Can you work these out from the model? Positions are in its coordinate system, mm. Face numbers are marked on the shaded views. A direction names the side the tool comes from. Coordinates: 2 decimals unless noted, no trailing zeros. Loops run counter-clockwise (first coordinate to the right, second up) from the corner with the lowest first, then second, coordinate; pieces in that order, holes last.
```python
from build123d import *

# Parameters (mm, degrees)
BOSS_EXTRUDE1_DEPTH                                 = 34
CBORE_FOR_M3_HEX_SOCKET_HEAD_CAP_SCREW1_D           = 3.4
CBORE_FOR_M3_HEX_SOCKET_HEAD_CAP_SCREW1_CBORE_D     = 6.5
CBORE_FOR_M3_HEX_SOCKET_HEAD_CAP_SCREW1_CBORE_DEPTH = 10


with BuildPart() as part:
    # Sketch1 → Boss-Extrude1 (new, symmetric)
    with BuildSketch(Plane.XY):
        Polygon((0, 0), (0, -11.547005384), (20, -11.547005384), align=None)
    extrude(amount=BOSS_EXTRUDE1_DEPTH, both=True)

    # CBORE for M3 Hex Socket Head Cap Screw1 (through all)
    with Locations(Plane(origin=(0, 0, 0), x_dir=(1, 0, 0), z_dir=(0, 1, 0))):
        with Locations((8, -25), (8, 25)):
            CounterBoreHole(CBORE_FOR_M3_HEX_SOCKET_HEAD_CAP_SCREW1_D / 2, CBORE_FOR_M3_HEX_SOCKET_HEAD_CAP_SCREW1_CBORE_D / 2, CBORE_FOR_M3_HEX_SOCKET_HEAD_CAP_SCREW1_CBORE_DEPTH)

    # Chamfer1
    # the kernel refuses this chamfer: 0.5, 0.366025404 mm, written as the material it takes off along each edge
    with BuildSketch(Plane(origin=(0.333333333, -11.21367205, 33.666666667), x_dir=(0.7071067811865475, -0.7071067811865476, 0), z_dir=(-0.5773502691896258, -0.5773502691896257, 0.5773502691896256)), Plane(origin=(0.333333333, -11.21367205, -33.666666667), x_dir=(0.7071067811865474, 0, -0.7071067811865476), z_dir=(-0.5773502691896258, -0.5773502691896257, -0.5773502691896257))) as chamfer1_piece_1:
        Polygon((-0.353553391, -0.204124145), (0.353553391, -0.204124145), (0, 0.40824829), align=None)
    extrude(amount=0.635085296, mode=Mode.SUBTRACT)
    with BuildSketch(Plane(origin=(19.105662433, -11.319334483, 33.666666667), x_dir=(-0.8880738339771186, 0.3250575836718637, 0.3250575836718637), z_dir=(0.25056280708572953, -0.2505628070857271, 0.9351131265310311))) as chamfer1_piece_2:
        Polygon((-0.478383292, 0.07914139), (1.059805709, 0.07914139), (-0.581422417, -0.15828278), align=None)
    extrude(amount=0.652121763, mode=Mode.SUBTRACT)
    with BuildSketch(Plane(origin=(19.105662433, -11.319334483, -33.666666667), x_dir=(0.8880738339771186, -0.3250575836718637, 0.3250575836718637), z_dir=(0.25056280708572953, -0.2505628070857271, -0.9351131265310311))) as chamfer1_piece_3:
        Polygon((-1.059805709, 0.07914139), (0.478383292, 0.07914139), (0.581422417, -0.15828278), align=None)
    extrude(amount=0.652121763, mode=Mode.SUBTRACT)
    with BuildSketch(Plane(origin=(0.311004234, -0.494016936, -33.666666667), x_dir=(0.5773502691896288, -0.5773502691896194, -0.5773502691896291), z_dir=(-0.16369153687076843, 0.6109051323707225, -0.7745966692414806))) as chamfer1_piece_4:
        Polygon((-0.349679369, 0.136409614), (0.516346035, 0.136409614), (-0.166666667, -0.272819228), align=None)
    extrude(amount=0.671995646, mode=Mode.SUBTRACT)
    with BuildSketch(Plane(origin=(0.311004234, -0.494016936, 33.666666667), x_dir=(0.5773502691896286, -0.5773502691896196, 0.5773502691896291), z_dir=(-0.1636915368707684, 0.6109051323707224, 0.7745966692414807))) as chamfer1_piece_5:
        Polygon((-0.349679369, -0.136409614), (0.516346035, -0.136409614), (-0.166666667, 0.272819228), align=None)
    extrude(amount=0.671995646, mode=Mode.SUBTRACT)
    with BuildSketch(Plane(origin=(-1.285841494, -11.547005384, 34), x_dir=(0, -0.02749587661058574, -0.9996219169112968), z_dir=(1, 0, 0)), Plane(origin=(-1.285841494, -11.547005384, -34), x_dir=(0, 0.999621916911297, -0.0274958766105822), z_dir=(1, 0, 0))) as chamfer1_piece_6:
        with BuildLine():
            Line((0.514336598, 0), (-0.028273577, 0.513558897))
            Line((-0.028273577, 0.513558897), (-0.038269797, 0.513283938))
            ThreePointArc((-0.038269797, 0.513283938), (-0.017064614, 0.256698915), (-0.009996219, -0.000274959))
            Line((-0.009996219, -0.000274959), (0.000274959, -0.009996219))
            ThreePointArc((0.000274959, -0.009996219), (0.257248832, -0.002927825), (0.514611556, -0.009996219))
            Line((0.514611556, -0.009996219), (0.514336598, 0))
        make_face()
    extrude(amount=22.571682988, mode=Mode.SUBTRACT)
    with BuildSketch(Plane(origin=(8, -11.547005384, -25), x_dir=(-1, 0, 0), z_dir=(0, 0, 1))) as chamfer1_piece_7:
        with BuildLine():
            Line((2.214142136, 0.014142136), (1.685857864, -0.514142136))
            Line((1.685857864, -0.514142136), (1.675857864, -0.514142136))
            ThreePointArc((1.675857864, -0.514142136), (1.69, -0.257071068), (1.69, 0))
            Line((1.69, 0), (1.7, 0.01))
            ThreePointArc((1.7, 0.01), (1.957071068, 0.01), (2.214142136, 0.024142136))
            Line((2.214142136, 0.024142136), (2.214142136, 0.014142136))
        make_face()
    revolve(axis=Axis((8, -11.547005384, -25), (0, -1, 0)), mode=Mode.SUBTRACT)
    with BuildSketch(Plane(origin=(8, -11.547005384, 25), x_dir=(-1, 0, 0), z_dir=(0, 0, 1))) as chamfer1_piece_8:
        with BuildLine():
            Line((2.214142136, 0.014142136), (1.685857864, -0.514142136))
            Line((1.685857864, -0.514142136), (1.675857864, -0.514142136))
            ThreePointArc((1.675857864, -0.514142136), (1.69, -0.257071068), (1.69, 0))
            Line((1.69, 0), (1.7, 0.01))
            ThreePointArc((1.7, 0.01), (1.957071068, 0.01), (2.214142136, 0.024142136))
            Line((2.214142136, 0.024142136), (2.214142136, 0.014142136))
        make_face()
    revolve(axis=Axis((8, -11.547005384, 25), (0, -1, 0)), mode=Mode.SUBTRACT)
    with BuildSketch(Plane(origin=(0, 1.285841494, -34), x_dir=(-0.027495876610586483, 0, 0.9996219169112968), z_dir=(0, -1, 0))) as chamfer1_piece_9:
        with BuildLine():
            Line((0.514336598, 0), (-0.028273577, -0.513558897))
            Line((-0.028273577, -0.513558897), (-0.038269797, -0.513283938))
            ThreePointArc((-0.038269797, -0.513283938), (-0.017064614, -0.256698915), (-0.009996219, 0.000274959))
            Line((-0.009996219, 0.000274959), (0.000274959, 0.009996219))
            ThreePointArc((0.000274959, 0.009996219), (0.257248832, 0.002927825), (0.514611556, 0.009996219))
            Line((0.514611556, 0.009996219), (0.514336598, 0))
        make_face()
    extrude(amount=14.118688372, mode=Mode.SUBTRACT)
    with BuildSketch(Plane(origin=(21.113571399, -12.189926131, -34), x_dir=(-0.4998109584556428, -0.8656979742248838, -0.027495876610582233), z_dir=(-0.8660254037844419, 0.4999999999999943, 0))) as chamfer1_piece_10:
        with BuildLine():
            Line((0.514336598, 0), (-0.028273577, 0.513558897))
            Line((-0.028273577, 0.513558897), (-0.038269797, 0.513283938))
            ThreePointArc((-0.038269797, 0.513283938), (-0.017064614, 0.256698915), (-0.009996219, -0.000274959))
            Line((-0.009996219, -0.000274959), (0.000274959, -0.009996219))
            ThreePointArc((0.000274959, -0.009996219), (0.257248832, -0.002927825), (0.514611556, -0.009996219))
            Line((0.514611556, -0.009996219), (0.514336598, 0))
        make_face()
    extrude(amount=25.665693756, mode=Mode.SUBTRACT)
    with BuildSketch(Plane(origin=(21.113571399, -12.189926131, 34), x_dir=(-0.4998109584556428, -0.8656979742248838, 0.027495876610582233), z_dir=(-0.8660254037844419, 0.4999999999999943, 0))) as chamfer1_piece_11:
        with BuildLine():
            Line((0.514336598, 0), (-0.028273577, -0.513558897))
            Line((-0.028273577, -0.513558897), (-0.038269797, -0.513283938))
            ThreePointArc((-0.038269797, -0.513283938), (-0.017064614, -0.256698915), (-0.009996219, 0.000274959))
            Line((-0.009996219, 0.000274959), (0.000274959, 0.009996219))
            ThreePointArc((0.000274959, 0.009996219), (0.257248832, 0.002927825), (0.514611556, 0.009996219))
            Line((0.514611556, 0.009996219), (0.514336598, 0))
        make_face()
    extrude(amount=25.665693756, mode=Mode.SUBTRACT)
    with BuildSketch(Plane(origin=(0, -11.547005384, -35.285841494), x_dir=(-0.02749587661058639, 0.9996219169112968, 0), z_dir=(0, 0, 1))) as chamfer1_piece_12:
        with BuildLine():
            Line((0.514336598, 0), (-0.028273577, -0.513558897))
            Line((-0.028273577, -0.513558897), (-0.038269797, -0.513283938))
            ThreePointArc((-0.038269797, -0.513283938), (-0.017064614, -0.256698915), (-0.009996219, 0.000274959))
            Line((-0.009996219, 0.000274959), (0.000274959, 0.009996219))
            ThreePointArc((0.000274959, 0.009996219), (0.257248832, 0.002927825), (0.514611556, 0.009996219))
            Line((0.514611556, 0.009996219), (0.514336598, 0))
        make_face()
    extrude(amount=70.571682988, mode=Mode.SUBTRACT)
    with BuildSketch(Plane(origin=(0, 1.285841494, 34), x_dir=(-0.027495876610586483, 0, -0.9996219169112968), z_dir=(0, -1, 0))) as chamfer1_piece_13:
        with BuildLine():
            Line((0.514336598, 0), (-0.028273577, 0.513558897))
            Line((-0.028273577, 0.513558897), (-0.038269797, 0.513283938))
            ThreePointArc((-0.038269797, 0.513283938), (-0.017064614, 0.256698915), (-0.009996219, -0.000274959))
            Line((-0.009996219, -0.000274959), (0.000274959, -0.009996219))
            ThreePointArc((0.000274959, -0.009996219), (0.257248832, -0.002927825), (0.514611556, -0.009996219))
            Line((0.514611556, -0.009996219), (0.514336598, 0))
        make_face()
    extrude(amount=14.118688372, mode=Mode.SUBTRACT)
    with BuildSketch(Plane(origin=(20, -11.547005384, 35.285841494), x_dir=(-0.9996219169112968, -0.02749587661058555, 0), z_dir=(0, 0, -1))) as chamfer1_piece_14:
        with BuildLine():
            Line((0.514336598, 0), (0.297309717, 0.20540729))
            Line((0.297309717, 0.20540729), (0.292073486, 0.21392679))
            ThreePointArc((0.292073486, 0.21392679), (0.148476438, 0.10299394), (-0.005236231, 0.0085195))
            Line((-0.005236231, 0.0085195), (0.000274959, -0.009996219))
            ThreePointArc((0.000274959, -0.009996219), (0.257248832, -0.002927825), (0.514611556, -0.009996219))
            Line((0.514611556, -0.009996219), (0.514336598, 0))
        make_face()
    extrude(amount=70.571682988, mode=Mode.SUBTRACT)
    with BuildSketch(Plane(origin=(0, 0, 35.285841494), x_dir=(-0.05197283076278021, -0.9986484991539833, 0), z_dir=(0, 0, -1))) as chamfer1_piece_15:
        with BuildLine():
            Line((0.371704143, 0), (0.220983806, -0.464444069))
            Line((0.220983806, -0.464444069), (0.212075392, -0.468987213))
            ThreePointArc((0.212075392, -0.468987213), (0.107882689, -0.233552691), (-0.008908414, -0.004543145))
            Line((-0.008908414, -0.004543145), (0.000519728, 0.009986485))
            ThreePointArc((0.000519728, 0.009986485), (0.185869781, 0.000340281), (0.372223871, 0.009986485))
            Line((0.372223871, 0.009986485), (0.371704143, 0))
        make_face()
    extrude(amount=70.571682988, mode=Mode.SUBTRACT)


solid = part.part
```
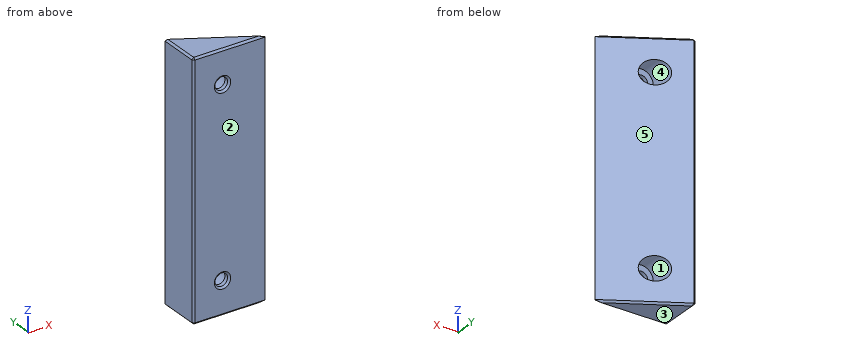
(1) I want a section at C-C on x = 8. Write out the boundary of the cut face in (y, z).
Check values:
outline: (-11.55, -33.5) - (-11.05, -34) - (-5.2, -34) - (-4.62, -33.5) - (-4.62, -28.25) - (-10, -28.25) - (-10, -26.7) - (-11.05, -26.7) - (-11.55, -27.2) - close; (-11.55, -22.8) - (-11.05, -23.3) - (-10, -23.3) - (-10, -21.75) - (-4.62, -21.75) - (-4.62, 21.75) - (-10, 21.75) - (-10, 23.3) - (-11.05, 23.3) - (-11.55, 22.8) - close; (-11.55, 27.2) - (-11.05, 26.7) - (-10, 26.7) - (-10, 28.25) - (-4.62, 28.25) - (-4.62, 33.5) - (-5.2, 34) - (-11.05, 34) - (-11.55, 33.5) - close
(2) Which directions (+Z, -Z, +X, -X, +Y, -Y) give clear straight access to the entire face, cutting with the end or side of a thin tool? Please do the marked faces 1 and 2.
Check values:
face 1: +Y
face 2: +Z, -Z, +X, -X, -Y
(3) I want a section at A-A on y = -8.25. Write out the boundary of the cut face in (x, z).
Check values:
outline: (0, -33.5) - (0.5, -34) - (13.29, -34) - (14.29, -33.5) - (14.29, 33.5) - (13.29, 34) - (0.5, 34) - (0, 33.5) - close; hole circle Ø6.5 at (8, -25); hole circle Ø6.5 at (8, 25)
(4) I'm going to push flat-ended pins straight in: pin 1 (1 mm diameter, centred on x = 6.5, z = -17, fed in from +Y); pin 2 (5 mm diameter, centred on x = 9, z = 24.5, fed in from +Y); pin 3 (4 mm diameter, centred on x = 8, z = 25, fed in from +Y). Where does each tip first touch, or does it pass through?
Check values:
pin 1: stops at y = -3.46
pin 2: stops at y = -5.36
pin 3: stops at y = -10
(5) If I drill on probe 1 along Z at (x, y) = (8, -8); probe 2 along Z at (x, y) = (8, -10.7); probe 3 along X at (y, z) = (-4.75, 25), over which ranges is the centre line in solid material (lowest first)?
Check values:
probe 1: z = -34 to -28.25, -21.75 to 21.75, 28.25 to 34
probe 2: z = -34 to -26.7, -23.3 to 23.3, 26.7 to 34
probe 3: x = 0 to 4.75
(6) I want a section at D-D on y = -3.5. Write out the boundary of the cut face in (x, z).
Check values:
outline: (0, -33.5) - (0.5, -34) - (5.06, -34) - (6.06, -33.5) - (6.06, -27.61) arc R3.25 cw to (6.06, -22.39) - (6.06, 22.39) arc R3.25 cw to (6.06, 27.61) - (6.06, 33.5) - (5.06, 34) - (0.5, 34) - (0, 33.5) - close
(7) If we mould it in two halves opening along X, with no side actions, what happens to the marked faces 3, 4 and 5? For each: released by +X, released by -X, zero draft, split by the parting line, or undercut.
Check values:
face 3: zero draft
face 4: undercut
face 5: released by +X
(8) I want a section at B-B on z = -25. Write out the boundary of the cut face in (x, y), then the cut area to 3 significant figures.
Check values:
outline: (0, -11.05) - (0.5, -11.55) - (5.8, -11.55) - (6.3, -11.05) - (6.3, -10) - (4.75, -10) - (4.75, -2.74) - (0.43, -0.25) - (0, -0.37) - close; (9.7, -11.05) - (10.2, -11.55) - (19.5, -11.55) - (19.68, -11.36) - (11.25, -6.5) - (11.25, -10) - (9.7, -10) - close
area: 74.7 mm2
